Design review of the part shown in the three views and the two pictorial views. Dimensions are in mm from the part's minimum x, y and z. A direction names the side the tool comes from. Round coordinates to 2 decimals unless told otherwise and drop trailing zeros. Loops run counter-clockwise (first coordinate to the right, second up) from the corner with the lowest first, then second, coordinate; pieces in that order, holes last.
1) Wall thickness on L1, parallel to Y at x = 57.15, z = 8.5; L2, parallel to X at y = 32, z = 4.5; L3, parallel to X at y = 22, z = 22.25: over which ranges is each line inside the solid? List them lowest first.
2) Take a section at B-B (z = 20.5). State the section outline as (x, y) points.
3) Take a section at C-C (y = 6.35). State the section outline as (x, z) points.
4) Mouldability with a two-part tool opening along X and no side actions: class the marked faces 1, 2, 3 and 4 as pulls with the +X half, pulls with the -X half, needs draft (parallel to the pull), parting line crosses it, or undercut.
5) Take a section at D-D (y = 27.5). State the section outline as (x, z) points, then the cut area to 3 significant figures.
6) Take a section at A-A (x = 6.35). State the section outline as (y, z) points.
7) Insertion check: pin 1 (3 mm diameter, centred on x = 57.15, y = 19.05, fed in from +Z); pin 2 (1.5 mm diameter, centred on x = 21, z = 6, fed in from -Y); pin 3 (19 mm diameter, centred on x = 32, y = 10, fed in from +Z). Each pin has a flat end and moves straight along its axis. Give the tip position at first contact, or say it passes through.
8) Tool access review of the marked faces 5 and 6: name each direction out of +Z, -Z, +X, -X, +Y, -Y from which nothing blocks a thin tool from reaching the whole face with its end or side.
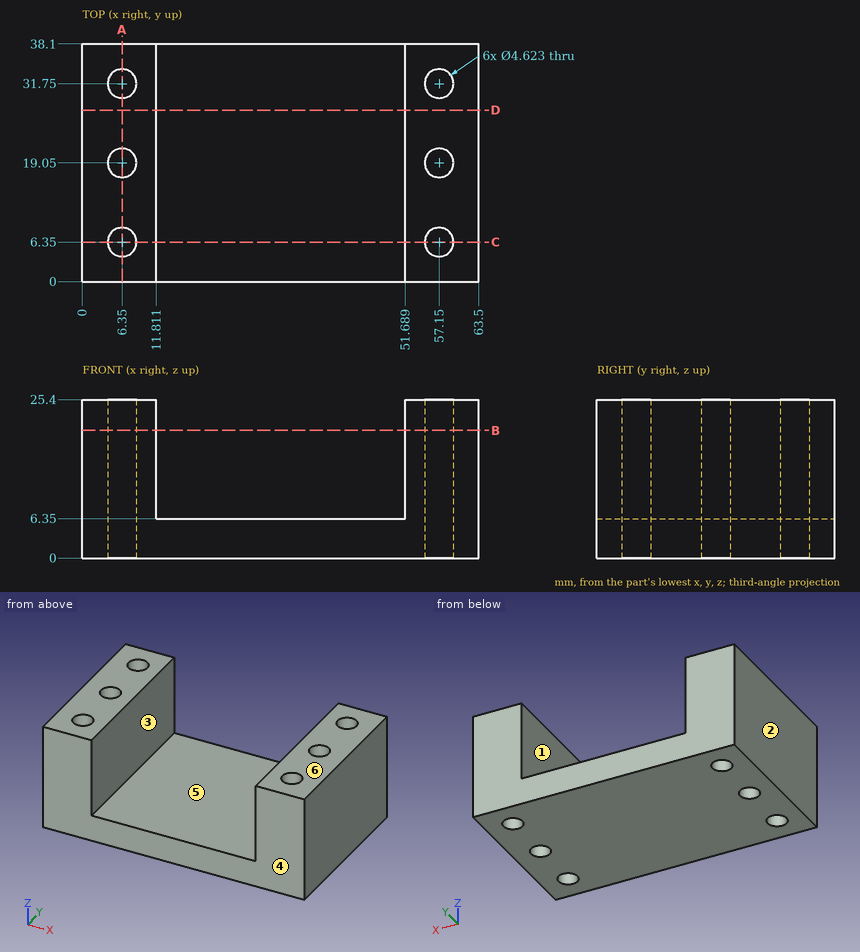
Response:
1. L1: y = 0 to 4.04, 8.66 to 16.74, 21.36 to 29.44, 34.06 to 38.1
1. L2: x = 0 to 4.05, 8.65 to 54.85, 59.45 to 63.5
1. L3: x = 0 to 11.81, 51.69 to 63.5
2. outline: (0, 0) - (11.81, 0) - (11.81, 38.1) - (0, 38.1) - close; (51.69, 0) - (63.5, 0) - (63.5, 38.1) - (51.69, 38.1) - close; hole circle Ø4.62 at (6.35, 6.35); hole circle Ø4.62 at (6.35, 19.05); hole circle Ø4.62 at (6.35, 31.75); hole circle Ø4.62 at (57.15, 6.35); hole circle Ø4.62 at (57.15, 19.05); hole circle Ø4.62 at (57.15, 31.75)
3. outline: (0, 0) - (4.04, 0) - (4.04, 25.4) - (0, 25.4) - close; (8.66, 0) - (54.84, 0) - (54.84, 25.4) - (51.69, 25.4) - (51.69, 6.35) - (11.81, 6.35) - (11.81, 25.4) - (8.66, 25.4) - close; (59.46, 0) - (63.5, 0) - (63.5, 25.4) - (59.46, 25.4) - close
4. face 1: undercut
4. face 2: pulls with the -X half
4. face 3: undercut
4. face 4: needs draft
5. outline: (0, 0) - (63.5, 0) - (63.5, 25.4) - (51.69, 25.4) - (51.69, 6.35) - (11.81, 6.35) - (11.81, 25.4) - (0, 25.4) - close
5. area: 853 mm2
6. outline: (0, 0) - (4.04, 0) - (4.04, 25.4) - (0, 25.4) - close; (8.66, 0) - (16.74, 0) - (16.74, 25.4) - (8.66, 25.4) - close; (21.36, 0) - (29.44, 0) - (29.44, 25.4) - (21.36, 25.4) - close; (34.06, 0) - (38.1, 0) - (38.1, 25.4) - (34.06, 25.4) - close
7. pin 1: passes through
7. pin 2: stops at y = 0
7. pin 3: stops at z = 6.35
8. face 5: +Z, +Y, -Y
8. face 6: +Z, +X, -X, +Y, -Y
